Verification items for the finished model (mm, model axes). A direction names the side the tool comes from. Round coordinates to 2 decimals unless told otherwise and drop trailing zeros. Order: outer loops, then holes, each group sorted by start corner. A loop starts at its lowest first (then second) coordinate and runs counter-clockwise, first axis right, second up. Notation, with made-up numbers: M -27,39 L 12,39 A6 ccw 12,46 Z; hole C 52.5,-12.75 d4. An arc over 180 degrees is marked long. Answer as a JSON object with one key per item and string values. Group by question number.
```python
from build123d import *

# Parameters (mm, degrees)
CROQUIS1_R              = 10.925
SALIENTE_EXTRUIR1_DEPTH = 3.6
CROQUIS2_R              = 1.775
CORTAR_EXTRUIR1_DEPTH   = 3.6
CROQUIS3_R              = 5.075
SALIENTE_EXTRUIR2_DEPTH = 10.15
SALIENTE_EXTRUIR3_START = 1.5
CROQUIS4_R              = 5.075
SALIENTE_EXTRUIR3_DEPTH = 1.5
CROQUIS5_R              = 3.575
CORTAR_EXTRUIR2_DEPTH   = 31.5
CHAFL_N1_SIZE           = 0.15


with BuildPart() as part:
    # Croquis1 → Saliente-Extruir1 (new body)
    with BuildSketch(Plane(origin=(0, 0, 0), x_dir=(1, 0, 0), z_dir=(0, 1, 0))):
        with Locations(Location((0, 0, 0), (0, 0, 270))):
            Circle(CROQUIS1_R)
    extrude(amount=SALIENTE_EXTRUIR1_DEPTH)

    # Croquis2 → Cortar-Extruir1 (cut)
    with BuildSketch(Plane(origin=(0, 3.6, 0), x_dir=(1, 0, 0), z_dir=(0, 1, 0))):
        with Locations(Location((-8.05, 0, 0), (0, 0, 270))):
            Circle(CROQUIS2_R)
        with Locations(Location((8.05, 0, 0), (0, 0, 270))):
            Circle(CROQUIS2_R)
        with Locations(Location((0, -8.05, 0), (0, 0, 270))):
            Circle(CROQUIS2_R)
        with Locations(Location((0, 8.05, 0), (0, 0, 270))):
            Circle(CROQUIS2_R)
    extrude(amount=-CORTAR_EXTRUIR1_DEPTH, mode=Mode.SUBTRACT)

    # Croquis3 → Saliente-Extruir2 (add)
    with BuildSketch(Plane(origin=(0, 3.6, 0), x_dir=(1, 0, 0), z_dir=(0, 1, 0))):
        with Locations(Location((0, 0, 0), (0, 0, 270))):
            Circle(CROQUIS3_R)
    extrude(amount=SALIENTE_EXTRUIR2_DEPTH)

    # Croquis4 → Saliente-Extruir3 (add)
    with BuildSketch(Plane.XZ.offset(SALIENTE_EXTRUIR3_START)):
        with Locations(Location((0, 0, 0), (0, 0, 90))):
            Circle(CROQUIS4_R)
    extrude(amount=-SALIENTE_EXTRUIR3_DEPTH)

    # Croquis5 → Cortar-Extruir2 (cut)
    with BuildSketch(Plane.XZ.offset(1.5)):
        with Locations(Location((0, 0, 0), (0, 0, 270))):
            Circle(CROQUIS5_R)
    extrude(amount=-CORTAR_EXTRUIR2_DEPTH, mode=Mode.SUBTRACT)

    # Chaflán1
    chafl_n1_edges = [part.edges().sort_by_distance(p)[0] for p in [
        (8.05, 0, -1.775),
        (8.05, 3.6, -1.775),
        (0, 0, 6.275),
        (0, 3.6, 6.275),
        (0, 0, -9.825),
        (0, 3.6, -9.825),
        (0, 0, -10.925),
        (0, 13.75, -5.075),
        (0, -1.5, -5.075),
        (0, 3.6, -10.925),
        (-8.05, 0, -1.775),
        (-8.05, 3.6, -1.775),
    ]]
    chamfer(chafl_n1_edges, length=CHAFL_N1_SIZE)


solid = part.part
```
Q1. Tool access check on faces 1 (the face through (-2, 3.6, 5)), 2 (the face through (0.078, 1.823, 6.277)). Record the directions out of +Z, -Z, +X, -X, +Y, -Y that give a thin tool (end or side, any length) a straight path to the whole face; none if there is none.
Q2. Release check for a two-part mould opening along Z. For faces 3 (the face through (-6.65, 1.78, -8.67)), 4 (the face through (-2, 0, 5)), 5 (the face through (3.545, 6.018, 0.465)) record: released by +Z, released by -Z, zero draft, split by the parting line, or undercut.
Q3. Thickness scan on line 1 (X direction, y = 2.3, z = 0) (3 decimals); line 2 (Y direction, x = 8, z = -3.25); line 3 (Z direction, x = -0.5, y = 12). Record the ranges inside material, lowest first. Write a range as from..to.
Q4. Gauge pin test, flat ends, axial feed: pin 1 Ø4.5 at (x, z) = (0, 8.05) entering from +Y; pin 2 Ø5.5 at (x, z) = (8.05, 0) entering from -Y; pin 3 Ø2 at (y, z) = (7.5, -1.5) entering from +X. Record the tip position at first contact, or that the pin passes through.
Q5. Cross-section at B-B, the plane z = 0. Give the number of separate pieces and of enclosed holes in the cut face, then the cut area to 3 significant figures.
Q6. Cross-section at A-A, the plane y = 11. Record the cut outline in (x, z) (3 decimals), then the cut area to 3 significant figures.
Conclusion:
{
 "1": {"face 1": "+Y", "face 2": "+Y, -Y"},
 "2": {"face 3": "split by the parting line", "face 4": "zero draft", "face 5": "undercut"},
 "3": {"line 1": "-10.925..-9.825, -6.275..-3.575, 3.575..6.275, 9.825..10.925", "line 2": "0..3.6", "line 3": "-5.05..-3.54, 3.54..5.05"},
 "4": {"pin 1": "y = 3.6", "pin 2": "y = 0", "pin 3": "x = 5.05"},
 "5": {"separate pieces": "4", "enclosed holes": "0", "area": "62.1 mm2"},
 "6": {"outline": "C 0,0 d10.15; hole C 0,0 d7.15", "area": "40.8 mm2"}
}
